Autodesk Inventor part; units mm, degrees
ref_plane "Płaszczyzna konstrukcyjna1" through (-11.5, -11.5, -2) normal (0, 0, -1) x (0, 1, 0)
ref_plane "YZ Plane" through (0, 0, 0) normal (1, 0, 0) x (0, 1, 0)
ref_plane "XZ Plane" through (0, 0, 0) normal (0, 1, 0) x (-1, 0, 0)
sketch "Szkic1" plane through (0, 0, 0) normal (0, 0, 1) x (1, 0, 0)
  circle A0 centre (0, 0) radius 17.5
  circle A1 centre (0, 0) radius 15
  line L0 (-3, -17.2409) -> (3, -17.2409)
  line L1 (3, -17.2409) -> (3, 17.2409)
  line L2 (3, 17.2409) -> (-3, 17.2409)
  line L3 (-3, 17.2409) -> (-3, -17.2409)
  line L4 (-3, -17.2409) -> (3, 17.2409) construction
  line L5 (3, -17.2409) -> (-3, 17.2409) construction
  line L6 (17.2409, 3) -> (-17.2409, 3)
  line L7 (-17.2409, 3) -> (-17.2409, -3)
  line L8 (-17.2409, -3) -> (17.2409, -3)
  line L9 (17.2409, -3) -> (17.2409, 3)
  line L10 (17.2409, 3) -> (-17.2409, -3) construction
  line L11 (-17.2409, 3) -> (17.2409, -3) construction
  circle A2 centre (0, 0) radius 1.75
  point P0 (-3, 3)
  point P1 (-3, -3)
  point P2 (3, -3)
  point P3 (3, 3)
  dimension "d0" = 6
  dimension "d1" = 6
  dimension "d2" = 3.5
extrude "Wyciągnięcie proste1" add sketch "Szkic1" along normal blind 3 contours L9 L8 A1 L6 | L1 A1 L3 L2 | A1 L8 L1 L6 | L0 L3 A1 L1 | L1 L6 L3 A1 | L1 L8 L3 L6 | A1 L3 L8 L1 | L6 A1 L8 L7 | L3 L8 A1 L6 | A2
sketch "Szkic2" plane through (0, 0, 3) normal (0, 0, 1) x (1, 0, 0)
  circle A0 centre (0, 0) radius 1.75
  dimension "d5" = 3.5
extrude "Wyciągnięcie proste2" cut sketch "Szkic2" against normal through all
sketch "Szkic3" plane through (0, 0, 0) normal (0, 0, -1) x (-1, 0, 0)
  circle A0 centre (0, 0) radius 1.75
  circle A1 centre (0, 0) radius 3.75
  dimension "d8" = 2
ref_plane "Płaszczyzna konstrukcyjna1" through (-11.5, -11.5, -2) normal (0, 0, -1) x (0, 1, 0)
extrude "Wyciągnięcie proste3" add sketch "Szkic3" along normal up to surface (2 mm away)
sketch "Szkic4" plane through (0, 0, 3) normal (0, 0, 1) x (1, 0, 0)
  circle A0 centre (0, 0) radius 17.5
  circle A1 centre (0, 0) radius 1.75
  line L0 (-17.2409, 3) -> (-17.2409, -3)
  line L1 (-17.2409, -3) -> (-3, -3)
  line L2 (-3, -3) -> (-3, -17.2409)
  line L3 (-3, -17.2409) -> (3, -17.2409)
  line L4 (3, -17.2409) -> (3, -3)
  line L5 (3, -3) -> (17.2409, -3)
  line L6 (17.2409, -3) -> (17.2409, 3)
  line L7 (17.2409, 3) -> (3, 3)
  line L8 (3, 3) -> (3, 17.2409)
  line L9 (3, 17.2409) -> (-3, 17.2409)
  line L10 (-3, 17.2409) -> (-3, 3)
  line L11 (-3, 3) -> (-17.2409, 3)
  line L12 (17.2409, 3) -> (3, 3)
  line L13 (17.2409, 3) -> (19.7409, 3)
  line L14 (19.7409, 3) -> (19.7409, -3)
  line L15 (19.7409, -3) -> (17.2409, -3)
  line L16 (17.2409, -3) -> (17.2409, 3)
  line L17 (-3, 3) -> (-17.2409, 3)
  line L18 (-17.2409, 3) -> (-19.7409, 3)
  line L19 (-19.7409, 3) -> (-19.7409, -3)
  line L20 (-19.7409, -3) -> (-17.2409, -3)
  line L21 (-17.2409, -3) -> (-17.2409, 3)
  line L22 (-3, -17.2409) -> (3, -17.2409)
  line L23 (3, -17.2409) -> (3, -19.7409)
  line L24 (3, -19.7409) -> (-3, -19.7409)
  line L25 (-3, -19.7409) -> (-3, -17.2409)
  line L26 (3, 17.2409) -> (-3, 17.2409)
  line L27 (-3, 17.2409) -> (-3, 19.7409)
  line L28 (-3, 19.7409) -> (3, 19.7409)
  line L29 (3, 19.7409) -> (3, 17.2409)
  dimension "d11" = 2.5
  dimension "d12" = 2.5
  dimension "d13" = 2.5
  dimension "d14" = 2.5
extrude "Wyciągnięcie proste4" add sketch "Szkic4" against normal blind 3 contours A0 L6 | A0 L13 L14 L15 | L9 A0 | A0 L27 L28 L29 | L23 L24 L25 A0 | A0 L3 | L0 A0 | A0 L20 L19 L18
sketch "Szkic5" plane through (0, 0, 0) normal (0, 0, -1) x (-1, 0, 0)
  circle A0 centre (0, 0) radius 17.5
  circle A1 centre (0, 0) radius 3.75
  line L0 (3, 3) -> (19.7409, 3)
  line L1 (3, 3) -> (3, 19.7409)
  line L2 (3, 19.7409) -> (-3, 19.7409)
  line L3 (-3, 3) -> (-3, 19.7409)
  line L4 (-3, 3) -> (-19.7409, 3)
  line L5 (-19.7409, 3) -> (-19.7409, -3)
  line L6 (-3, -3) -> (-19.7409, -3)
  line L7 (-3, -3) -> (-3, -19.7409)
  line L8 (-3, -19.7409) -> (3, -19.7409)
  line L9 (3, -3) -> (3, -19.7409)
  line L10 (3, -3) -> (19.7409, -3)
  line L11 (19.7409, -3) -> (19.7409, 3)
  circle A2 centre (0, 0) radius 17.7
  point P0 (3, -17.4439)
  point P1 (-3, -17.4439)
  point P2 (17.4439, 3)
  point P3 (17.4439, -3)
  point P4 (-17.4439, -3)
  point P5 (-17.4439, 3)
  point P6 (-3, 17.4439)
  point P7 (3, 17.4439)
  dimension "d17" = 0.2
extrude "Wyciągnięcie proste5" add sketch "Szkic5" along normal blind 1.5 contours L0 L11 L10 A2 | A2 L3 L2 L1 | L9 L8 L7 A2 | A2 L6 L5 L4
fillet "Zaokrąglenie1" radius 2 19 edges at (-3, -3, 1.5) (-3, -19.7409, 1.5) (-3, -19.7409, -0.75) (-19.7409, -3, -0.75) (-19.7409, -3, 1.5) (3, -19.7409, -0.75) (3, -19.7409, 1.5) (3, -3, 1.5) (19.7409, -3, 1.5) (19.7409, -3, -0.75) (19.7409, 3, -0.75) (19.7409, 3, 1.5) (3, 3, 1.5) (3, 19.7409, 1.5) (3, 19.7409, -0.75) (-3, 19.7409, -0.75) (-3, 19.7409, 1.5) (-19.7409, 3, 1.5) (-19.7409, 3, -0.75)
fillet "Zaokrąglenie2" radius 2 1 edges at (-3, 3, 1.5)
sketch "Szkic6" plane through (0, 0, 0) normal (0, 0, -1) x (-1, 0, 0)
  circle A0 centre (0, 0) radius 17.5
  arc A1 (17.4439, -3) -> (17.4439, 3) centre (0, 0) ccw
  line L0 (5, 3) -> (17.4439, 3)
  arc A2 (3, 5) -> (5, 3) centre (5, 5) ccw
  line L1 (3, 5) -> (3, 17.4439)
  arc A3 (3, 17.4439) -> (-3, 17.4439) centre (0, 0) ccw
  line L2 (-3, 5) -> (-3, 17.4439)
  arc A4 (-5, 3) -> (-3, 5) centre (-5, 5) ccw
  line L3 (-5, 3) -> (-17.4439, 3)
  arc A5 (-17.4439, 3) -> (-17.4439, -3) centre (0, 0) ccw
  line L4 (-5, -3) -> (-17.4439, -3)
  arc A6 (-3, -5) -> (-5, -3) centre (-5, -5) ccw
  line L5 (-3, -5) -> (-3, -17.4439)
  arc A7 (-3, -17.4439) -> (3, -17.4439) centre (0, 0) ccw
  line L6 (3, -5) -> (3, -17.4439)
  arc A8 (5, -3) -> (3, -5) centre (5, -5) ccw
  line L7 (5, -3) -> (17.4439, -3)
  circle A9 centre (0, 0) radius 3.75
  point P0 (3, -17.2409)
  point P1 (-3, -17.2409)
  point P2 (-17.2409, -3)
  point P3 (-17.2409, 3)
  point P4 (-3, 17.2409)
  point P5 (3, 17.2409)
  point P6 (17.2409, 3)
  point P7 (17.2409, -3)
  dimension "d22" = 35
extrude "Wyciągnięcie proste6" add sketch "Szkic6" along normal up to surface (1.5 mm away) contours A0 L0 A1 L7 | A0 L2 A3 L1 | L6 A7 L5 A0 | A0 L4 A5 L3
properties part number "gora"
Check sheet for the modelled part. Datum: model origin and axes. Units: mm. A direction names the side the tool comes from. Round coordinates to 2 decimals unless told otherwise and drop trailing zeros. Loops run counter-clockwise (first coordinate to the right, second up) from the corner with the lowest first, then second, coordinate; pieces in that order, holes last.
1. Sectioned sample at B-B on x = 0. Record the boundary of the cut face in (y, z).
2. Set-up check for faces 5 (the flat face through (3, 11, 2)), 6 (the flat face through (0, -18, -1.5)), 7 (the flat face through (-3, 3, 0)): record each of +Z, -Z, +X, -X, +Y, -Y from which the full face is reachable in a straight line by a thin tool's end or side.
3. Sectioned sample at A-A on z = -0.65. Record the boundary of the cut face in (x, y).
4. Mould release check, pull along X, two halves, no side actions. Record for faces 1 (the cylindrical face through (3.746, -0.165, -0.986)), 2 (the cylindrical face through (0, -17.5, -0.7)), 3 (the cylindrical face through (19.17, 2.4, 0.78)), 4 (the flat face through (19, 0, -1.5)): released by +X, released by -X, zero draft, split by the parting line, or undercut.
5. Sectioned sample at D-D on z = 2.4. Record the boundary of the cut face in (x, y).
6. Scan lines: probe 1 along Y at (x, z) = (0, 2); probe 2 along X at (y, z) = (14, 1.3). Record each from-to range of solid material in increasing order.
7. Gauge pin test, flat ends, axial feed: pin 1 Ø2.5 at (x, y) = (-18, 0) entering from -Z; pin 2 Ø2 at (y, z) = (-13, 0) entering from +X; pin 3 Ø2 at (x, z) = (-2.5, 2) entering from +Y. Record the tip position at first contact, or that the pin passes through.
Recorded:
1. outline: (-19.74, -1.5) - (-17.5, -1.5) - (-17.5, 0) - (-3.75, 0) - (-3.75, -2) - (-1.75, -2) - (-1.75, 3) - (-19.74, 3) - close; (1.75, -2) - (3.75, -2) - (3.75, 0) - (17.5, 0) - (17.5, -1.5) - (19.74, -1.5) - (19.74, 3) - (1.75, 3) - close
2. face 5: +Z, -Z, +X, +Y
2. face 6: -Z, +X, -X, -Y
2. face 7: -Z
3. outline: (-19.74, -1) arc R2 ccw to (-17.74, -3) - (-17.24, -3) arc R17.5 cw to (-17.24, 3) - (-17.74, 3) arc R2 ccw to (-19.74, 1) - close; circle Ø7.5 at (0, 0); (-3, -17.74) arc R2 ccw to (-1, -19.74) - (1, -19.74) arc R2 ccw to (3, -17.74) - (3, -17.24) arc R17.5 cw to (-3, -17.24) - close; (-3, 17.24) arc R17.5 cw to (3, 17.24) - (3, 17.74) arc R2 ccw to (1, 19.74) - (-1, 19.74) arc R2 ccw to (-3, 17.74) - close; (17.24, -3) - (17.74, -3) arc R2 ccw to (19.74, -1) - (19.74, 1) arc R2 ccw to (17.74, 3) - (17.24, 3) arc R17.5 cw to start; hole circle Ø3.5 at (0, 0)
4. face 1: undercut
4. face 2: undercut
4. face 3: released by +X
4. face 4: zero draft
5. outline: (-19.74, -1) arc R2 ccw to (-17.74, -3) - (-5, -3) arc R2 cw to (-3, -5) - (-3, -17.74) arc R2 ccw to (-1, -19.74) - (1, -19.74) arc R2 ccw to (3, -17.74) - (3, -5) arc R2 cw to (5, -3) - (17.74, -3) arc R2 ccw to (19.74, -1) - (19.74, 1) arc R2 ccw to (17.74, 3) - (5, 3) arc R2 cw to (3, 5) - (3, 17.74) arc R2 ccw to (1, 19.74) - (-1, 19.74) arc R2 ccw to (-3, 17.74) - (-3, 5) arc R2 cw to (-5, 3) - (-17.74, 3) arc R2 ccw to (-19.74, 1) - close; hole circle Ø3.5 at (0, 0)
6. probe 1: y = -19.74 to -1.75, 1.75 to 19.74
6. probe 2: x = -3 to 3
7. pin 1: stops at z = -1.5
7. pin 2: stops at x = 3
7. pin 3: stops at y = 19.68
